Read the model definition and answer for the solid it produces. Units are mm, in the model's axes. A direction names the side the tool comes from. Give positions to 0.01 mm unless a question says otherwise; leave off trailing zeros. Order: outer loops, then holes, each group sorted by start corner. A loop starts at its lowest first (then second) coordinate and runs counter-clockwise, first axis right, second up. Notation, with made-up numbers: (78.25, 0) -> (125.25, 0) arc R23 ccw to (125.25, 11) -> close; hole circle Ø2 at (-26.5, 74). An arc over 180 degrees is marked (long way). Use one line per item in the form item = value.
```python
from build123d import *

# Parameters (mm, degrees)
SKETCH1_W           = 169.5
SKETCH1_H           = 97.5
BASE_DEPTH          = 1.7
MOUNTHOLES_REACH    = 99.786
SKETCH2_R           = 1.5
SKETCH3_W           = 12.51
SKETCH3_H           = 31
SKETCH3_W_2         = 69.6
SKETCH3_H_2         = 12.51
DSUBMAIN_DEPTH      = 12.6
SKETCH4_R           = 2.4
BOSS_EXTRUDE3_DEPTH = 5.5
SKETCH5_R           = 2.4
BOSS_EXTRUDE4_DEPTH = 5.5
SKETCH6_R           = 2.4
BOSS_EXTRUDE5_DEPTH = 5.5
BOSS_EXTRUDE6_START = 5.5
SKETCH7_R           = 2.4
BOSS_EXTRUDE6_DEPTH = 5.5
SKETCH8_W           = 5.5
SKETCH8_H           = 8
USB_DEPTH           = 3
SKETCH9_W           = 2.3
SKETCH9_H           = 1.26
LED_DEPTH           = 1
SKETCH10_W          = 2.5
SKETCH10_H          = 2.5
BOSS_EXTRUDE9_DEPTH = 9


with BuildPart() as part:
    # Sketch1 → Base (new body)
    with BuildSketch(Plane(origin=(0, 0, 0), x_dir=(1, 0, 0), z_dir=(0, 1, 0))):
        Rectangle(SKETCH1_W, SKETCH1_H)
    extrude(amount=BASE_DEPTH)

    # Sketch2 → MountHoles (cut, up to next)
    with BuildSketch(Plane(origin=(0, 1.7, 0), x_dir=(1, 0, 0), z_dir=(0, 1, 0)), mode=Mode.PRIVATE) as mountholes_sk1:
        with Locations(Location((82.21, 46.21, 0), (0, 0, 270))):
            Circle(SKETCH2_R)
    mountholes_tool1 = extrude(mountholes_sk1.sketch, amount=-MOUNTHOLES_REACH, mode=Mode.PRIVATE) & part.part
    # Sketch2 → MountHoles (cut, up to next)
    with BuildSketch(Plane(origin=(0, 1.7, 0), x_dir=(1, 0, 0), z_dir=(0, 1, 0)), mode=Mode.PRIVATE) as mountholes_sk2:
        with Locations(Location((82.21, -46.21, 0), (0, 0, 270))):
            Circle(SKETCH2_R)
    mountholes_tool2 = extrude(mountholes_sk2.sketch, amount=-MOUNTHOLES_REACH, mode=Mode.PRIVATE) & part.part
    # Sketch2 → MountHoles (cut, up to next)
    with BuildSketch(Plane(origin=(0, 1.7, 0), x_dir=(1, 0, 0), z_dir=(0, 1, 0)), mode=Mode.PRIVATE) as mountholes_sk3:
        with Locations(Location((-69.51, -45.57, 0), (0, 0, 270))):
            Circle(SKETCH2_R)
    mountholes_tool3 = extrude(mountholes_sk3.sketch, amount=-MOUNTHOLES_REACH, mode=Mode.PRIVATE) & part.part
    # Sketch2 → MountHoles (cut, up to next)
    with BuildSketch(Plane(origin=(0, 1.7, 0), x_dir=(1, 0, 0), z_dir=(0, 1, 0)), mode=Mode.PRIVATE) as mountholes_sk4:
        with Locations(Location((-82.21, 46.21, 0), (0, 0, 270))):
            Circle(SKETCH2_R)
    mountholes_tool4 = extrude(mountholes_sk4.sketch, amount=-MOUNTHOLES_REACH, mode=Mode.PRIVATE) & part.part
    add(mountholes_tool1.solids().sort_by_distance((82.21, 1.7, -46.21))[0], mode=Mode.SUBTRACT)
    add(mountholes_tool2.solids().sort_by_distance((82.21, 1.7, 46.21))[0], mode=Mode.SUBTRACT)
    add(mountholes_tool3.solids().sort_by_distance((-69.51, 1.7, 45.57))[0], mode=Mode.SUBTRACT)
    add(mountholes_tool4.solids().sort_by_distance((-82.21, 1.7, -46.21))[0], mode=Mode.SUBTRACT)

    # Sketch3 → DSUBMain (add)
    with BuildSketch(Plane(origin=(0, 1.7, 0), x_dir=(1, 0, 0), z_dir=(0, 1, 0))):
        with Locations((-80.145, 1.59)):
            Rectangle(SKETCH3_W, SKETCH3_H)
        with Locations((-80.145, -33.35)):
            Rectangle(SKETCH3_W, SKETCH3_H)
        with Locations((80.145, 2.72)):
            Rectangle(SKETCH3_W, SKETCH3_H)
        with Locations((16.18, 44.195)):
            Rectangle(SKETCH3_W_2, SKETCH3_H_2)
        with Locations((16.18, -44.195)):
            Rectangle(SKETCH3_W_2, SKETCH3_H_2)
    extrude(amount=DSUBMAIN_DEPTH)

    # Sketch4 → Boss-Extrude3 (add)
    with BuildSketch(Plane(origin=(86.4, 0, 0), x_dir=(0, 0, -1), z_dir=(1, 0, 0))):
        with Locations(Location((-8.73, 8, 0), (0, 0, 180))):
            Circle(SKETCH4_R)
        with Locations(Location((14.17, 8, 0), (0, 0, 180))):
            Circle(SKETCH4_R)
        Polygon((-6.28, 11.8), (11.72, 11.8), (10.22, 4.2), (-4.78, 4.2), align=None)
    extrude(amount=BOSS_EXTRUDE3_DEPTH)

    # Sketch5 → Boss-Extrude4 (add)
    with BuildSketch(Plane.ZY.offset(86.4)):
        with Locations(Location((-13.04, 8, 0), (0, 0, 180))):
            Circle(SKETCH5_R)
        with Locations(Location((9.86, 8, 0), (0, 0, 180))):
            Circle(SKETCH5_R)
        with Locations(Location((21.9, 8, 0), (0, 0, 180))):
            Circle(SKETCH5_R)
        with Locations(Location((44.8, 8, 0), (0, 0, 180))):
            Circle(SKETCH5_R)
        Polygon((-10.59, 11.8), (7.41, 11.8), (5.91, 4.2), (-9.09, 4.2), align=None)
        Polygon((24.35, 11.8), (42.35, 11.8), (40.85, 4.2), (25.85, 4.2), align=None)
    extrude(amount=BOSS_EXTRUDE4_DEPTH)

    # Sketch6 → Boss-Extrude5 (add)
    with BuildSketch(Plane.XY.offset(50.45)):
        with Locations(Location((-15.57, 8, 0), (0, 0, 180))):
            Circle(SKETCH6_R)
        with Locations(Location((47.93, 8, 0), (0, 0, 180))):
            Circle(SKETCH6_R)
        Polygon((-11.22, 11.8), (43.58, 11.8), (42.08, 4.2), (-9.72, 4.2), align=None)
    extrude(amount=BOSS_EXTRUDE5_DEPTH)

    # Sketch7 → Boss-Extrude6 (add)
    with BuildSketch(Plane(origin=(0, 0, -50.45), x_dir=(-1, 0, 0), z_dir=(0, 0, -1)).offset(BOSS_EXTRUDE6_START)):
        with Locations((-47.93, 8)):
            Circle(SKETCH7_R)
        with Locations((15.57, 8)):
            Circle(SKETCH7_R)
        Polygon((11.22, 11.8), (-43.58, 11.8), (-42.08, 4.2), (9.72, 4.2), align=None)
    extrude(amount=-BOSS_EXTRUDE6_DEPTH)

    # Sketch8 → USB (add)
    with BuildSketch(Plane(origin=(0, 1.7, 0), x_dir=(1, 0, 0), z_dir=(0, 1, 0))):
        with Locations((-83.1, 28.19)):
            Rectangle(SKETCH8_W, SKETCH8_H)
    extrude(amount=USB_DEPTH)

    # Sketch9 → LED (add)
    with BuildSketch(Plane(origin=(0, 1.7, 0), x_dir=(1, 0, 0), z_dir=(0, 1, 0))):
        with Locations((-82.8, 41.47)):
            Rectangle(SKETCH9_W, SKETCH9_H)
        with Locations((-82.8, 35.75)):
            Rectangle(SKETCH9_W, SKETCH9_H)
        with Locations((-82.8, 22.57)):
            Rectangle(SKETCH9_W, SKETCH9_H)
        with Locations((-82.8, 20.03)):
            Rectangle(SKETCH9_W, SKETCH9_H)
    extrude(amount=LED_DEPTH)

    # Sketch10 → Boss-Extrude9 (add)
    with BuildSketch(Plane(origin=(0, 1.7, 0), x_dir=(1, 0, 0), z_dir=(0, 1, 0))):
        with Locations((71.33, 40.08)):
            Rectangle(SKETCH10_W, SKETCH10_H)
        with Locations((71.33, 27.47)):
            Rectangle(SKETCH10_W, SKETCH10_H)
    extrude(amount=BOSS_EXTRUDE9_DEPTH)


solid = part.part
```
Item 1: Which of the six approach directions +Z, -Z, +X, -X, +Y, -Y give full straight-line access (tool end or side, diameter ignored) to faces 1 (the flat face through (-80, 8, 13.91)), 2 (the flat face through (80, 8, 12.78)), 3 (the flat face through (-10.46, 7.95, -53.24)), 4 (the flat face through (-89, 11.8, 33)), 5 (the cylindrical face through (-17.86, 7.28, 53.16))?
Checks:
face_1 = +X, -X, +Y
face_2 = +Z, +X, +Y
face_3 = -Z, -Y
face_4 = +Z, -Z, -X, +Y
face_5 = +Z
Item 2: The part is cut by section B-B on x = 47.93. Give the vertices of the cut face in (y, z).
Checks:
outline = (0, -48.75) -> (1.7, -48.75) -> (1.7, -50.45) -> (5.6, -50.45) -> (5.6, -55.95) -> (10.4, -55.95) -> (10.4, -50.45) -> (14.3, -50.45) -> (14.3, -37.94) -> (1.7, -37.94) -> (1.7, 37.94) -> (14.3, 37.94) -> (14.3, 50.45) -> (10.4, 50.45) -> (10.4, 55.95) -> (5.6, 55.95) -> (5.6, 50.45) -> (1.7, 50.45) -> (1.7, 48.75) -> (0, 48.75) -> close
Item 3: The part is cut by section D-D on z = 1. Give the vertices of the cut face in (x, y), and give its area (3 significant figures).
Checks:
outline = (-91.9, 4.2) -> (-86.4, 4.2) -> (-86.4, 1.7) -> (-84.75, 1.7) -> (-84.75, 0) -> (84.75, 0) -> (84.75, 1.7) -> (86.4, 1.7) -> (86.4, 4.2) -> (91.9, 4.2) -> (91.9, 11.8) -> (86.4, 11.8) -> (86.4, 14.3) -> (73.89, 14.3) -> (73.89, 1.7) -> (-73.89, 1.7) -> (-73.89, 14.3) -> (-86.4, 14.3) -> (-86.4, 11.8) -> (-91.9, 11.8) -> close
area = 687 mm²
Item 4: The part is cut by section A-A on z = 28. Give the vertices of the cut face in (x, y).
Checks:
outline = (-91.9, 4.2) -> (-86.4, 4.2) -> (-86.4, 1.7) -> (-84.75, 1.7) -> (-84.75, 0) -> (84.75, 0) -> (84.75, 1.7) -> (-73.89, 1.7) -> (-73.89, 14.3) -> (-86.4, 14.3) -> (-86.4, 11.8) -> (-91.9, 11.8) -> close
Item 5: The part is cut by section C-C on y = 8. State how many separate pieces and enclosed holes the cut face has, and give its area (3 significant figures).
Checks:
separate_pieces = 7
enclosed_holes = 0
area = 4,040 mm²
Item 6: Straight lines are drawn through the part: L1, parallel to Z at x = 82.21, y = 0.35; L2, parallel to X at y = 0.4, z = -46.21; L3, parallel to Z at x = -82.21, y = 1.45. For each, find the intervals that lie inside material, in ascending order. Write a range as from..to.
Checks:
L1 = -48.75..-47.71, -44.71..44.71, 47.71..48.75
L2 = -84.75..-83.71, -80.71..80.71, 83.71..84.75
L3 = -48.75..-47.71, -44.71..48.75
Item 7: Given pin 1 Ø2 at (x, y) = (-59, 2) entering from -Z; pin 2 Ø3 at (x, y) = (72, 5) entering from +Z; pin 3 Ø0.5 at (x, z) = (18, -50) entering from -Y; pin 4 Ø8 at (x, y) = (-18, 3.5) entering from -Z, each flat-ended and moving along its own axis, determine where each tip first touches the part or whether it passes through.
Checks:
pin_1 = -48.75
pin_2 = -26.22
pin_3 = 1.7
pin_4 = -55.95
